Design review of the part built by this model. Coordinates are the model's own, in mm. A direction names the side the tool comes from. Coordinates: 2 decimals unless noted, no trailing zeros. Write each loop counter-clockwise with the first axis right and the second up, starting at its lowest first coordinate (ties: lowest second). Pieces come first, ordered by that corner, then holes. Notation, with made-up numbers: M 11.5,0 L 40.5,0 A20 cw 40.5,9 Z; hole C -19,14 d3. An arc over 180 degrees is marked long. Return JSON: item names as keys, results as strings. Group by question number.
```python
from build123d import *

# Parameters (mm, degrees)
SKETCH_5_W          = 55
SKETCH_5_H          = 3
EXTRUDE_1_DEPTH     = 5
CUT_EXTRUDE_1_REACH = 57.308
SKETCH_6_R          = 1.6
CUT_EXTRUDE_2_REACH = 57.308
SKETCH_7_R          = 0.9
FILLET_1_R          = 1.5
SKETCH_8_W          = 6
SKETCH_8_H          = 1.6
CUT_EXTRUDE_3_DEPTH = 10
SKETCH_9_W          = 2.616592429
SKETCH_9_H          = 0.2
CUT_EXTRUDE_4_DEPTH = 10
SKETCH_10_R         = 1.6
SKETCH_10_R_2       = 0.9
EXTRUDE_2_DEPTH     = 0.5
EXTRUDE_START       = 0.5
SKETCH_11_R         = 0.9
SKETCH_11_R_2       = 1.6
EXTRUDE_3_DEPTH     = 0.5


with BuildPart() as part:
    # 草图5 → 凸台-拉伸1 (new body)
    with BuildSketch(Plane(origin=(0, 0, 0), x_dir=(1, 0, 0), z_dir=(0, 1, 0))):
        with Locations((27.5, -1.5)):
            Rectangle(SKETCH_5_W, SKETCH_5_H)
    extrude(amount=EXTRUDE_1_DEPTH)

    # 草图6 → 切除-拉伸1 (cut, up to next)
    with BuildSketch(Plane.XY.offset(3), mode=Mode.PRIVATE) as cut_extrude_1_sk1:
        with Locations((2.5, 2.5)):
            Circle(SKETCH_6_R)
    cut_extrude_1_tool1 = extrude(cut_extrude_1_sk1.sketch, amount=-CUT_EXTRUDE_1_REACH, mode=Mode.PRIVATE) & part.part
    add(cut_extrude_1_tool1.solids().sort_by_distance((2.5, 2.5, 3))[0], mode=Mode.SUBTRACT)

    # 草图7 → 切除-拉伸2 (cut, up to next)
    with BuildSketch(Plane.XY, mode=Mode.PRIVATE) as cut_extrude_2_sk1:
        with Locations(Location((53, 2.5, 0), (0, 0, 180))):
            Circle(SKETCH_7_R)
    cut_extrude_2_tool1 = extrude(cut_extrude_2_sk1.sketch, amount=CUT_EXTRUDE_2_REACH, mode=Mode.PRIVATE) & part.part
    add(cut_extrude_2_tool1.solids().sort_by_distance((53, 2.5, 0))[0], mode=Mode.SUBTRACT)

    # 圆角1
    fillet_1_edges = [part.edges().sort_by_distance(p)[0] for p in [
        (55, 5, 1.5),
        (55, 0, 1.5),
        (0, 0, 1.5),
        (0, 5, 1.5),
    ]]
    fillet(fillet_1_edges, radius=FILLET_1_R)

    # 草图8 → 切除-拉伸3 (cut)
    with BuildSketch(Plane(origin=(0, 5, 0), x_dir=(1, 0, 0), z_dir=(0, 1, 0))):
        with Locations((52, -1.5)):
            Rectangle(SKETCH_8_W, SKETCH_8_H)
    extrude(amount=-CUT_EXTRUDE_3_DEPTH, mode=Mode.SUBTRACT)

    # 草图9 → 切除-拉伸4 (cut)
    with BuildSketch(Plane.XZ):
        with Locations((50.308296215, 0.6)):
            Rectangle(SKETCH_9_W, SKETCH_9_H)
        with Locations((50.308296215, 2.4)):
            Rectangle(SKETCH_9_W, SKETCH_9_H)
    extrude(amount=-CUT_EXTRUDE_4_DEPTH, mode=Mode.SUBTRACT)

    # 草图10 → 凸台-拉伸2 (add)
    with BuildSketch(Plane.XY.offset(3)):
        with BuildLine():
            Line((55, 1.5), (55, 3.5))
            ThreePointArc((55, 3.5), (54.560660172, 4.560660172), (53.5, 5))
            Line((53.5, 5), (1.5, 5))
            ThreePointArc((1.5, 5), (0.439339828, 4.560660172), (0, 3.5))
            Line((0, 3.5), (0, 1.5))
            ThreePointArc((0, 1.5), (0.439339828, 0.439339828), (1.5, 0))
            Line((1.5, 0), (53.5, 0))
            ThreePointArc((53.5, 0), (54.560660172, 0.439339828), (55, 1.5))
        make_face()
        with Locations((2.5, 2.5)):
            Circle(SKETCH_10_R, mode=Mode.SUBTRACT)
        with Locations((53, 2.5)):
            Circle(SKETCH_10_R_2, mode=Mode.SUBTRACT)
    extrude(amount=EXTRUDE_2_DEPTH)

    # 草图11 → 凸台-拉伸3 (add)
    with BuildSketch(Plane(origin=(0, 0, 0), x_dir=(-1, 0, 0), z_dir=(0, 0, -1)).offset(EXTRUDE_START)):
        with BuildLine():
            Line((-1.5, 5), (-53.5, 5))
            ThreePointArc((-53.5, 5), (-54.560660172, 4.560660172), (-55, 3.5))
            Line((-55, 3.5), (-55, 1.5))
            ThreePointArc((-55, 1.5), (-54.560660172, 0.439339828), (-53.5, 0))
            Line((-53.5, 0), (-1.5, 0))
            ThreePointArc((-1.5, 0), (-0.439339828, 0.439339828), (0, 1.5))
            Line((0, 1.5), (0, 3.5))
            ThreePointArc((0, 3.5), (-0.439339828, 4.560660172), (-1.5, 5))
        make_face()
        with Locations(Location((-53, 2.5, 0), (0, 0, 180))):
            Circle(SKETCH_11_R, mode=Mode.SUBTRACT)
        with Locations(Location((-2.5, 2.5, 0), (0, 0, 180))):
            Circle(SKETCH_11_R_2, mode=Mode.SUBTRACT)
    extrude(amount=-EXTRUDE_3_DEPTH)


solid = part.part
```
Item 1: For pin 1 (2.5 mm diameter, centred on x = 53, y = 2.5, fed in from +Z), flat-tipped, find the tip position at first contact; note if it passes through.
Item 2: Add section D-D (z = 1.5). Write out the cut boundary in (x, y), plus the area to 3 significant figures.
Item 3: Machinability: for faces 5 (the flat face through (50, 2, 0.5)), 6 (the flat face through (54, 3, 0.7)), 7 (the flat face through (0, 2, 1)), which of the approach directions +Z, -Z, +X, -X, +Y, -Y give a long, thin tool a straight path to every point of the face, cutting with its end or side? Answer none if there is none.
Item 4: The part is to be moulded in two halves that separate along Z. For faces 1 (the flat face through (27, 3, 3.5)), 2 (the flat face through (54, 3, 2.3)), 3 (the flat face through (50, 2, 2.5)), 4 (the flat face through (27, 5, 1)), say which applies: pulls with the +Z half, pulls with the -Z half, needs draft (parallel to the pull), parting line crosses it, or undercut.
Item 5: Add section C-C (x = 2.5). Write out the cut boundary in (y, z), plus the area to 3 significant figures.
Item 6: For line 1 (X direction, y = 2.6, z = 2.85); line 2 (Y direction, x = 2.5, z = 1.7); line 3 (Y direction, x = 53, z = 0.25), list the stretches that pass through material, from the lowest coordinate up.
Item 7: Add section B-B (y = 2.5). Write out the cut boundary in (x, z).
Geometry check:
{
 "1": {"pin 1": "z = 3.5"},
 "2": {"outline": "M 0,1.5 A1.5 ccw 1.5,0 L 49,0 L 49,5 L 1.5,5 A1.5 ccw 0,3.5 Z; hole C 2.5,2.5 d3.2", "area": "236 mm^2"},
 "3": {"face 5": "+Y, -Y", "face 6": "+X, +Y, -Y", "face 7": "+Z, -Z, -X, +Y, -Y"},
 "4": {"face 1": "pulls with the +Z half", "face 2": "undercut", "face 3": "undercut", "face 4": "needs draft"},
 "5": {"outline": "M 0,-0.5 L 0.9,-0.5 L 0.9,3.5 L 0,3.5 Z; M 4.1,-0.5 L 5,-0.5 L 5,3.5 L 4.1,3.5 Z", "area": "7.20 mm^2"},
 "6": {"line 1": "0 to 0.9, 4.1 to 52.11, 53.89 to 55", "line 2": "0 to 0.9, 4.1 to 5", "line 3": "0 to 1.6, 3.4 to 5"},
 "7": {"outline": "M 0,-0.5 L 0.9,-0.5 L 0.9,3.5 L 0,3.5 Z; M 4.1,-0.5 L 52.1,-0.5 L 52.1,0.7 L 51.62,0.7 L 51.62,0.5 L 49,0.5 L 49,2.5 L 51.62,2.5 L 51.62,2.3 L 52.1,2.3 L 52.1,3.5 L 4.1,3.5 Z; M 53.9,-0.5 L 55,-0.5 L 55,0.7 L 53.9,0.7 Z; M 53.9,2.3 L 55,2.3 L 55,3.5 L 53.9,3.5 Z"}
}
